from build123d import *

# Parameters (mm, degrees)
SKETCH_3_R      = 1.5
SKETCH_3_R_2    = 2
SKETCH_3_R_3    = 24.001454592
SKETCH_3_R_4    = 20
SKETCH_3_W      = 7.2
SKETCH_3_H      = 2.2
SKETCH_3_W_2    = 8.2
EXTRUDE_1_DEPTH = 2


with BuildPart() as part:
    # 草图3 → 凸台-拉伸1 (new body)
    with BuildSketch(Plane.XY):
        with BuildLine():
            Line((-46.5, 360.009783315), (-46.5, 310.009783315))
            Line((-46.5, 310.009783315), (-49.5, 310.009783315))
            Line((-49.5, 310.009783315), (-49.5, 305.009783315))
            Line((-49.5, 305.009783315), (-46.5, 305.009783315))
            Line((-46.5, 305.009783315), (-46.5, 300.009783315))
            Line((-46.5, 300.009783315), (-44, 300.009783315))
            Line((-44, 300.009783315), (-44, 301.509783315))
            Line((-44, 301.509783315), (-41.4, 301.509783315))
            Line((-41.4, 301.509783315), (-41.4, 300.009783315))
            Line((-41.4, 300.009783315), (-38.4, 300.009783315))
            Line((-38.4, 300.009783315), (-38.4, 297.009783315))
            Line((-38.4, 297.009783315), (-41.4, 297.009783315))
            Line((-41.4, 297.009783315), (-41.4, 295.509783315))
            Line((-41.4, 295.509783315), (-44, 295.509783315))
            Line((-44, 295.509783315), (-44, 297.009783315))
            Line((-44, 297.009783315), (-46.5, 297.009783315))
            Line((-46.5, 297.009783315), (-46.5, 295.009783315))
            Line((-46.5, 295.009783315), (-49.5, 295.009783315))
            Line((-49.5, 295.009783315), (-49.5, 290.009783315))
            Line((-49.5, 290.009783315), (-46.5, 290.009783315))
            Line((-46.5, 290.009783315), (-46.5, 280.009783315))
            ThreePointArc((-46.5, 280.009783315), (-20.448024821, 150.009783315), (-46.5, 20.009783315))
            Line((-46.5, 20.009783315), (-49.5, 20.009783315))
            Line((-49.5, 20.009783315), (-49.5, 15.009783315))
            Line((-49.5, 15.009783315), (-46.5, 15.009783315))
            Line((-46.5, 15.009783315), (-46.5, 10.009783315))
            Line((-46.5, 10.009783315), (-44, 10.009783315))
            Line((-44, 10.009783315), (-44, 11.509783315))
            Line((-44, 11.509783315), (-41.4, 11.509783315))
            Line((-41.4, 11.509783315), (-41.4, 10.009783315))
            Line((-41.4, 10.009783315), (-38.4, 10.009783315))
            Line((-38.4, 10.009783315), (-38.4, 7.009783315))
            Line((-38.4, 7.009783315), (-41.4, 7.009783315))
            Line((-41.4, 7.009783315), (-41.4, 5.509783315))
            Line((-41.4, 5.509783315), (-44, 5.509783315))
            Line((-44, 5.509783315), (-44, 7.009783315))
            Line((-44, 7.009783315), (-46.5, 7.009783315))
            Line((-46.5, 7.009783315), (-46.5, 5.009783315))
            Line((-46.5, 5.009783315), (-49.5, 5.009783315))
            Line((-49.5, 5.009783315), (-49.5, 0.009783315))
            Line((-49.5, 0.009783315), (-46.5, 0.009783315))
            Line((-46.5, 0.009783315), (-46.5, -3.990216685))
            Line((-46.5, -3.990216685), (-26.5, -3.990216685))
            Line((-26.5, -3.990216685), (-26.5, 3.009783315))
            Line((-26.5, 3.009783315), (26.5, 3.009783315))
            Line((26.5, 3.009783315), (26.5, -3.990216685))
            Line((26.5, -3.990216685), (46.5, -3.990216685))
            Line((46.5, -3.990216685), (46.5, 0.009783315))
            Line((46.5, 0.009783315), (49.5, 0.009783315))
            Line((49.5, 0.009783315), (49.5, 5.009783315))
            Line((49.5, 5.009783315), (46.5, 5.009783315))
            Line((46.5, 5.009783315), (46.5, 7.009783315))
            Line((46.5, 7.009783315), (44, 7.009783315))
            Line((44, 7.009783315), (44, 5.509783315))
            Line((44, 5.509783315), (41.4, 5.509783315))
            Line((41.4, 5.509783315), (41.4, 7.009783315))
            Line((41.4, 7.009783315), (38.4, 7.009783315))
            Line((38.4, 7.009783315), (38.4, 10.009783315))
            Line((38.4, 10.009783315), (41.4, 10.009783315))
            Line((41.4, 10.009783315), (41.4, 11.509783315))
            Line((41.4, 11.509783315), (44, 11.509783315))
            Line((44, 11.509783315), (44, 10.009783315))
            Line((44, 10.009783315), (46.5, 10.009783315))
            Line((46.5, 10.009783315), (46.5, 15.009783315))
            Line((46.5, 15.009783315), (49.5, 15.009783315))
            Line((49.5, 15.009783315), (49.5, 20.009783315))
            Line((49.5, 20.009783315), (46.5, 20.009783315))
            ThreePointArc((46.5, 20.009783315), (20.448024821, 150.009783315), (46.5, 280.009783315))
            Line((46.5, 280.009783315), (46.5, 290.009783315))
            Line((46.5, 290.009783315), (49.5, 290.009783315))
            Line((49.5, 290.009783315), (49.5, 295.009783315))
            Line((49.5, 295.009783315), (46.5, 295.009783315))
            Line((46.5, 295.009783315), (46.5, 297.009783315))
            Line((46.5, 297.009783315), (44, 297.009783315))
            Line((44, 297.009783315), (44, 295.509783315))
            Line((44, 295.509783315), (41.4, 295.509783315))
            Line((41.4, 295.509783315), (41.4, 297.009783315))
            Line((41.4, 297.009783315), (38.4, 297.009783315))
            Line((38.4, 297.009783315), (38.4, 300.009783315))
            Line((38.4, 300.009783315), (41.4, 300.009783315))
            Line((41.4, 300.009783315), (41.4, 301.509783315))
            Line((41.4, 301.509783315), (44, 301.509783315))
            Line((44, 301.509783315), (44, 300.009783315))
            Line((44, 300.009783315), (46.5, 300.009783315))
            Line((46.5, 300.009783315), (46.5, 305.009783315))
            Line((46.5, 305.009783315), (49.5, 305.009783315))
            Line((49.5, 305.009783315), (49.5, 310.009783315))
            Line((49.5, 310.009783315), (46.5, 310.009783315))
            Line((46.5, 310.009783315), (46.5, 330.009783315))
            Line((46.5, 330.009783315), (34.06116735, 336.162324196))
            ThreePointArc((34.06116735, 336.162324196), (-11.38853896, 316.756491321), (-37.576612526, 358.666477673))
            Line((-37.576612526, 358.666477673), (-46.5, 360.009783315))
        make_face()
        with Locations((-31.5, -0.990216685)):
            Circle(SKETCH_3_R, mode=Mode.SUBTRACT)
        with Locations((31.5, -0.990216685)):
            Circle(SKETCH_3_R, mode=Mode.SUBTRACT)
        with Locations((0, 310.509783315)):
            Circle(SKETCH_3_R_2, mode=Mode.SUBTRACT)
        with Locations((-30.0520382, 322.957745114)):
            Circle(SKETCH_3_R_2, mode=Mode.SUBTRACT)
        with Locations((-42.5, 353.009783315)):
            Circle(SKETCH_3_R_2, mode=Mode.SUBTRACT)
        with Locations((30.0520382, 322.957745114)):
            Circle(SKETCH_3_R_2, mode=Mode.SUBTRACT)
        with Locations((0, 258.344771167)):
            Circle(SKETCH_3_R_3, mode=Mode.SUBTRACT)
        with Locations((0, 56.478199566)):
            Circle(SKETCH_3_R_4, mode=Mode.SUBTRACT)
        with Locations((0, 19.74399144)):
            Circle(SKETCH_3_R, mode=Mode.SUBTRACT)
        with Locations((0, 295.428004537)):
            Circle(SKETCH_3_R, mode=Mode.SUBTRACT)
        with Locations((-39, -0.990216685)):
            Rectangle(SKETCH_3_W, SKETCH_3_H, mode=Mode.SUBTRACT)
        with Locations((39, -0.990216685)):
            Rectangle(SKETCH_3_W, SKETCH_3_H, mode=Mode.SUBTRACT)
        with BuildLine():
            Line((-9.475517085, 113.355875718), (-9.475517085, 203.355875718))
            ThreePointArc((-9.475517085, 203.355875718), (0, 212.831392803), (9.475517085, 203.355875718))
            Line((9.475517085, 203.355875718), (9.475517085, 113.355875718))
            ThreePointArc((9.475517085, 113.355875718), (0, 103.880358633), (-9.475517085, 113.355875718))
        make_face(mode=Mode.SUBTRACT)
        with Locations((0, 90.179279099)):
            Rectangle(SKETCH_3_W_2, SKETCH_3_H, mode=Mode.SUBTRACT)
        with Locations((0, 223.587354689)):
            Rectangle(SKETCH_3_W_2, SKETCH_3_H, mode=Mode.SUBTRACT)
    extrude(amount=EXTRUDE_1_DEPTH)


solid = part.part
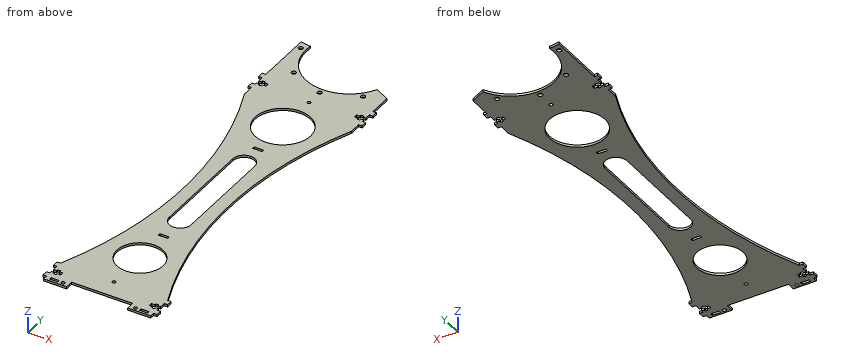
The listing builds one solid part. Answer for the finished solid, in the listing's coordinates (mm). Give positions to 0.01 mm unless a question says otherwise; leave off trailing zeros. Write each loop counter-clockwise with the first axis right and the second up, starting at its lowest first coordinate (ties: lowest second). Pieces come first, ordered by that corner, then holes. Notation, with made-up numbers: (25, -2.75) - (84, -2.75) arc R37 cw to (84, 33.25) - close; hole circle Ø5 at (88.5, -3.75). An arc over 180 degrees is marked (long way). One line per question, with ' | ' between items. Start each with the question number.
1. Section C-C, the plane z = 1.5 is taken. Count the separate pieces of the cut face and the enclosed holes in it, then the cut area to 3 significant figures.
2. Straight lines are drawn through the part: line 1 (X direction, y = 301, z = 0.3); line 2 (X direction, y = 146.5, z = 1.35); line 3 (Y direction, x = -10.5, z = 0.5). For each, find the intervals that lie inside material, in ascending order.
3. Section B-B, the plane y = 130.5 is taken. Determine the outline of the cut face in (x, z).
4. Section A-A, the plane y = 42 is taken. Determine the outline of the cut face in (x, z), then the cut area to 3 significant figures.
5. Given P1, Ø1, axis at x = 2, z = 1, coming from the -Y side; P2, Ø1, axis at x = -27.5, z = 1.5, coming from the +Y side; P3, Ø24, axis at x = 0, y = 56.48, coming from the -Z side; P4, Ø0.6, axis at x = 40, z = 0.5, coming from the +Y side, each flat-ended and moving along its own axis, determine where each tip first touches the part or whether it passes through.
Result:
1) separate pieces: 1 | enclosed holes: 15 | area: 16,100 mm2
2) line 1: x = -46.5 to -44, -41.4 to 41.4, 44 to 46.5 | line 2: x = -20.47 to -9.48, 9.48 to 20.47 | line 3: y = 3.01 to 39.46, 73.5 to 236.76, 279.93 to 316.49
3) outline: (-21.01, 0) - (-9.48, 0) - (-9.48, 2) - (-21.01, 2) - close; (9.48, 0) - (21.01, 0) - (21.01, 2) - (9.48, 2) - close
4) outline: (-38.2, 0) - (-13.8, 0) - (-13.8, 2) - (-38.2, 2) - close; (13.8, 0) - (38.2, 0) - (38.2, 2) - (13.8, 2) - close | area: 97.6 mm2
5) P1: stops at y = 3.01 | P2: stops at y = 327.32 | P3: passes through | P4: stops at y = 333.37
